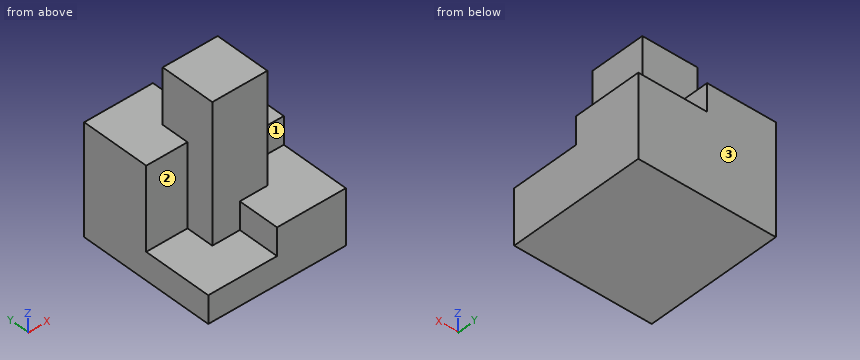
```python
from build123d import *

# Parameters (mm, degrees)
F1_DEPTH  = 20.32
F2_DEPTH  = 15.24
F3_DEPTH  = 25.4
F4_DEPTH  = 10.16
F3_FACE_W = 10.16
F3_FACE_H = 10.16
F5_DEPTH  = 5.08


with BuildPart() as f1:
    # F0 (on Top) → F1 (new body)
    with BuildSketch(Plane.XY):
        Polygon((0.808182, 12.730596), (-9.351818, 12.730596), (-11.891818, 12.730596), (-11.891818, 10.190596), (-11.891818, 0.030596), (-4.271818, 0.030596), (-4.271818, 5.110596), (0.808182, 5.110596), align=None)
    extrude(amount=F1_DEPTH)

    # F0 (on Top) → F2 (join)
    with BuildSketch(Plane.XY):
        Polygon((10.968182, 12.730596), (0.808182, 12.730596), (0.808182, 5.110596), (5.888182, 5.110596), (5.888182, 0.030596), (13.508182, 0.030596), (13.508182, 10.190596), (13.508182, 12.730596), align=None)
    extrude(amount=F2_DEPTH)

    # F0 (on Top) → F3 (join)
    with BuildSketch(Plane.XY):
        Polygon((5.888182, 5.110596), (0.808182, 5.110596), (-4.271818, 5.110596), (-4.271818, 0.030596), (-4.271818, -5.049404), (0.808182, -5.049404), (5.888182, -5.049404), (5.888182, 0.030596), align=None)
    extrude(amount=F3_DEPTH)

    # F0 (on Top) → F4 (join)
    with BuildSketch(Plane.XY):
        Polygon((13.508182, 0.030596), (5.888182, 0.030596), (5.888182, -5.049404), (0.808182, -5.049404), (0.808182, -12.669404), (10.968182, -12.669404), (13.508182, -12.669404), (13.508182, -10.129404), align=None)
    extrude(amount=F4_DEPTH)

    # F0 (on Top) + F3_face (on face) → F5 (join)
    with BuildSketch(Plane.XY):
        Polygon((-4.271818, 0.030596), (-11.891818, 0.030596), (-11.891818, -10.129404), (-11.891818, -12.669404), (-9.351818, -12.669404), (0.808182, -12.669404), (0.808182, -5.049404), (-4.271818, -5.049404), align=None)
    with BuildSketch(Plane(origin=(0.808182, 0.030596, 25.4), x_dir=(1, 0, 0), z_dir=(0, 0, 1))):
        Rectangle(F3_FACE_W, F3_FACE_H)
    extrude(amount=F5_DEPTH)


solid = f1.part
```
Geometry check sheet. Reference: the model listing, model coordinates, mm. Face numbers are marked on the shaded views. A direction names the side the tool comes from. Coordinates: 2 decimals unless noted, no trailing zeros. Order: outer loops, then holes, each group sorted by start corner. A loop starts at its lowest first (then second) coordinate and runs counter-clockwise, first axis right, second up.
Item 1: Section check C-C (y = -8.25). Enter the section's corners in (x, z).
Item 2: Depth check by flat-ended pin: pin 1 (11 mm diameter, centred on x = 0.5, z = 14.5, fed in from -Y); pin 2 (2.5 mm diameter, centred on x = 10, z = 12.5, fed in from -Y); pin 3 (5.5 mm diameter, centred on y = -9, z = 8.5, fed in from -X); pin 4 (12 mm diameter, centred on x = -7.5, z = 18, fed in from -Y). Enter the tip coordinate at first touch or a pass-through.
Item 3: Scan lines: line 1 along Z through (x, y) = (9.5, -1); line 2 along Y through (x, z) = (1, 17.5); line 3 along Z through (x, y) = (8.5, 9.5). Record each from-to range of solid material in increasing order.
Item 4: Section check B-B (z = 17). Enter the section's corners in (x, y).
Item 5: Section check A-A (x = 5.5). Enter the section's corners in (y, z), plus the area to 3 significant figures.
Item 6: Section check D-D (x = 11.75). Enter the section's corners in (y, z).
Item 7: Tool access check on the marked faces 1, 2 and 3. Record the directions out of +Z, -Z, +X, -X, +Y, -Y that give a thin tool (end or side, any length) a straight path to the whole face; none if there is none.
Check sheet entries:
1. outline: (-11.89, 0) - (13.51, 0) - (13.51, 10.16) - (0.81, 10.16) - (0.81, 5.08) - (-11.89, 5.08) - close
2. pin 1: stops at y = -12.67
2. pin 2: stops at y = 0.03
2. pin 3: stops at x = 0.81
2. pin 4: stops at y = -5.05
3. line 1: z = 0 to 10.16
3. line 2: y = -5.05 to 5.11
3. line 3: z = 0 to 15.24
4. outline: (-11.89, 0.03) - (-4.27, 0.03) - (-4.27, -5.05) - (5.89, -5.05) - (5.89, 5.11) - (0.81, 5.11) - (0.81, 12.73) - (-11.89, 12.73) - close
5. outline: (-12.67, 0) - (12.73, 0) - (12.73, 15.24) - (5.11, 15.24) - (5.11, 30.48) - (-5.05, 30.48) - (-5.05, 10.16) - (-12.67, 10.16) - close
5. area: 503 mm2
6. outline: (-12.67, 0) - (12.73, 0) - (12.73, 15.24) - (0.03, 15.24) - (0.03, 10.16) - (-12.67, 10.16) - close
7. face 1: +Z, +X, -Y
7. face 2: +Z, -X, -Y
7. face 3: +Z, -Z, +X, -X, +Y
